Design review of the part built by this model. Coordinates are the model's own, in mm. Round coordinates to 2 decimals unless told otherwise and drop trailing zeros. Write each loop counter-clockwise with the first axis right and the second up, starting at its lowest first coordinate (ties: lowest second). Pieces come first, ordered by that corner, then holes.
from build123d import *

# Parameters (mm, degrees)
SKETCH1_R           = 76.2
SKETCH1_R_2         = 5.08
BOSS_EXTRUDE1_DEPTH = 12.7
CHAMFER1_SIZE       = 13.198227154
CHAMFER1_SIZE_2     = 7.62
SKETCH3_R           = 5.08
BOSS_EXTRUDE2_DEPTH = 2.54
SKETCH4_R           = 4.064
BOSS_EXTRUDE3_DEPTH = 1.27
SKETCH5_R           = 4.572
BOSS_EXTRUDE4_DEPTH = 6.35


with BuildPart() as part:
    # Sketch1 → Boss-Extrude1 (new body)
    with BuildSketch(Plane.XY):
        Circle(SKETCH1_R)
        with Locations((38.1, 0)):
            Circle(SKETCH1_R_2, mode=Mode.SUBTRACT)
        with Locations((19.05, -32.995567884)):
            Circle(SKETCH1_R_2, mode=Mode.SUBTRACT)
        with Locations((-19.05, -32.995567884)):
            Circle(SKETCH1_R_2, mode=Mode.SUBTRACT)
        with Locations((-38.1, 0)):
            Circle(SKETCH1_R_2, mode=Mode.SUBTRACT)
        with Locations((-19.05, 32.995567884)):
            Circle(SKETCH1_R_2, mode=Mode.SUBTRACT)
        with Locations((19.05, 32.995567884)):
            Circle(SKETCH1_R_2, mode=Mode.SUBTRACT)
    extrude(amount=BOSS_EXTRUDE1_DEPTH)

    # Chamfer1
    # the kernel refuses this chamfer: 13.198227154, 7.62 mm, written as the material it takes off along each edge
    with BuildSketch(Plane(origin=(0, 0, 0), x_dir=(1, 0, 0), z_dir=(0, -1, 0))) as chamfer1_piece_1:
        Polygon((76.2, CHAMFER1_SIZE), (76.2 - CHAMFER1_SIZE_2, 0), (76.2, 0), align=None)
    revolve(axis=Axis((0, 0, 0), (0, 0, 1)), mode=Mode.SUBTRACT)

    # Sketch3 → Boss-Extrude2 (add)
    with BuildSketch(Plane(origin=(0, 0, 0), x_dir=(-1, 0, 0), z_dir=(0, 0, -1))):
        with Locations(Location((0, 0, 0), (0, 0, 180))):
            Circle(SKETCH3_R)
    extrude(amount=BOSS_EXTRUDE2_DEPTH)

    # Sketch4 → Boss-Extrude3 (add)
    with BuildSketch(Plane(origin=(0, 0, -2.54), x_dir=(-1, 0, 0), z_dir=(0, 0, -1))):
        Circle(SKETCH4_R)
    extrude(amount=BOSS_EXTRUDE3_DEPTH)

    # Sketch5 → Boss-Extrude4 (add)
    with BuildSketch(Plane(origin=(0, 0, -3.81), x_dir=(-1, 0, 0), z_dir=(0, 0, -1))):
        Circle(SKETCH5_R)
    extrude(amount=BOSS_EXTRUDE4_DEPTH)


solid = part.part
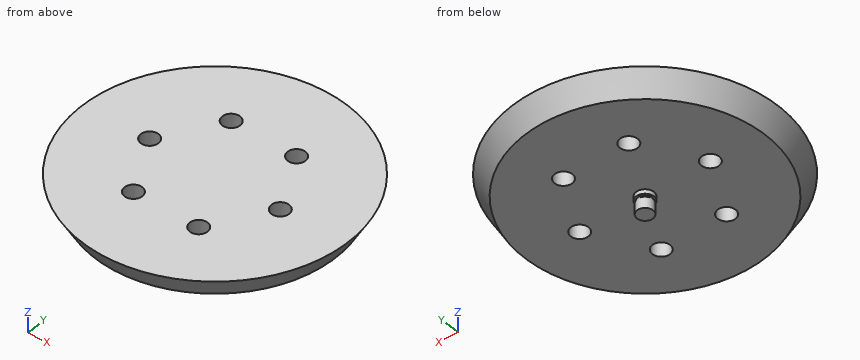
1) For P1, Ø16.5, axis at x = -19.05, y = 33, coming from the -Z side; P2, Ø1, axis at x = 20.5, z = 3, coming from the +Y side; P3, Ø2, axis at x = 0.5, z = 5, coming from the +Y side; P4, Ø9, axis at x = 19.05, y = -33, coming from the +Z side, all flat-tipped, find the tip position at first contact; note any pin that passes through.
2) Add section C-C on z = 6.75. State the section outline as (x, y) points, and give its area (3 significant figures).
3) For line 1 along Y through (x, z) = (-19.5, 4); line 2 along Y through (x, z) = (-19.05, 3.25); line 3 along X through (y, z) = (-37, 9.75), list the stretches that pass through material, from the lowest coordinate up.
4) Add section D-D on x = 19.05. Count the separate pieces of the cut face and the enclosed holes in it, and give its area (3 significant figures).
5) Add section B-B on x = 0. State the section outline as (y, z) points.
6) Add section A-A on y = 0. State the section outline as (x, z) points, and give its area (3 significant figures).
Computed:
1. P1: stops at z = 0
1. P2: stops at y = 67.59
1. P3: stops at y = 72.04
1. P4: passes through
2. outline: circle Ø144.95 at (0, 0); hole circle Ø10.16 at (-38.1, 0); hole circle Ø10.16 at (-19.05, -33); hole circle Ø10.16 at (-19.05, 33); hole circle Ø10.16 at (19.05, -33); hole circle Ø10.16 at (19.05, 33); hole circle Ø10.16 at (38.1, 0)
2. area: 16,000 mm2
3. line 1: y = -68.15 to -38.06, -27.94 to 27.94, 38.06 to 68.15
3. line 2: y = -67.83 to -38.08, -27.92 to 27.92, 38.08 to 67.83
3. line 3: x = -64.33 to -22.18, -15.92 to 15.92, 22.18 to 64.33
4. separate pieces: 3
4. enclosed holes: 0
4. area: 1,510 mm2
5. outline: (-75.91, 12.7) - (-68.58, 0) - (-5.08, 0) - (-5.08, -2.54) - (-4.06, -2.54) - (-4.06, -3.81) - (-4.57, -3.81) - (-4.57, -10.16) - (4.57, -10.16) - (4.57, -3.81) - (4.06, -3.81) - (4.06, -2.54) - (5.08, -2.54) - (5.08, 0) - (68.58, 0) - (75.91, 12.7) - close
6. outline: (-75.91, 12.7) - (-68.58, 0) - (-43.18, 0) - (-43.18, 12.7) - close; (-33.02, 0) - (-5.08, 0) - (-5.08, -2.54) - (-4.06, -2.54) - (-4.06, -3.81) - (-4.57, -3.81) - (-4.57, -10.16) - (4.57, -10.16) - (4.57, -3.81) - (4.06, -3.81) - (4.06, -2.54) - (5.08, -2.54) - (5.08, 0) - (33.02, 0) - (33.02, 12.7) - (-33.02, 12.7) - close; (43.18, 0) - (68.58, 0) - (75.91, 12.7) - (43.18, 12.7) - close
6. area: 1,670 mm2
